```python
from build123d import *

# Parameters (mm, degrees)
PAD_DEPTH       = 22
BOX_W           = 28
BOX_H           = 44
BOX_DEPTH       = 11
SKETCH001_R     = 8.75
POCKET_DEPTH    = 33
FILLET_R        = 2
SKETCH003_R     = 3
POCKET002_DEPTH = 28.001


with BuildPart() as part:
    # Sketch → Pad (new body)
    with BuildSketch(Plane.XY):
        Polygon((0, 1), (17, 1), (17, 10), (17.5, 10), (17.5, 22), (15, 25), (2, 25), (-0.5, 22), (-0.5, 10), (0, 10), align=None)
    extrude(amount=PAD_DEPTH)

    # Box → Box (join)
    with BuildSketch(Plane(origin=(-5.5, -10, 22), x_dir=(1, 0, 0), z_dir=(0, 0, 1))):
        with Locations((14, 22)):
            Rectangle(BOX_W, BOX_H)
    extrude(amount=BOX_DEPTH)

    # Sketch001 (on Face4 of Box) → Pocket (cut)
    with BuildSketch(Plane(origin=(-5.5, -10, 0), x_dir=(1, 0, 0), z_dir=(0, 0, -1))):
        with Locations((14, -24.5)):
            Circle(SKETCH001_R)
    extrude(amount=-POCKET_DEPTH, mode=Mode.SUBTRACT)

    # Fillet
    fillet_edges = [part.edges().sort_by_distance(p)[0] for p in [
        (17.5, 22, 11),
        (15, 25, 11),
        (2, 25, 11),
        (17, 1, 11),
        (0, 1, 11),
        (-0.5, 22, 11),
    ]]
    fillet(fillet_edges, radius=FILLET_R)

    # Sketch003 (on Face23 of Fillet) → Pocket002 (cut, through all)
    with BuildSketch(Plane(origin=(22.5, -10, 22), x_dir=(0, 1, 0), z_dir=(1, 0, 0))):
        with Locations((7, 5.5)):
            Circle(SKETCH003_R)
        with Locations((37, 5.5)):
            Circle(SKETCH003_R)
    extrude(amount=-POCKET002_DEPTH, mode=Mode.SUBTRACT)


solid = part.part
```
Input: part model. Units: mm. Frame: model coordinates. A direction names the side the tool comes from. Give positions to 0.01 mm unless a question says otherwise; leave off trailing zeros. Write each loop counter-clockwise with the first axis right and the second up, starting at its lowest first coordinate (ties: lowest second). Pieces come first, ordered by that corner, then holes. Notation, with made-up numbers: (28, -37) - (69, -37) arc R19 cw to (69, -32) - close; hole circle Ø7 at (11, 21.25). An arc over 180 degrees is marked (long way). Write item = value, one per line. Start each with the question number.
1) Cut plane C-C (x = 8.5). Return loops of the section in (y, z), and give its area (3 significant figures).
2) Draft query along Z for faces 6 (the face through (8, 1, 11)), 7 (the face through (15, 7, 33)), 8 (the face through (8.7, -5.4, 25.7)). Return one class per face: pulls with the +Z half, pulls with the -Z half, needs draft (parallel to the pull), parting line crosses it, or undercut.
3) Material intervals for L1, parallel to Y at x = 8.5, z = 28; L2, parallel to Y at x = 8.5, z = 7; L3, parallel to Y at x = 21, z = 25.5, sorted ascending. Write a range as [from, to].
4) Reachability of faces 1 (the face through (16.328, 23.406, 10.846)), 2 (the face through (9, 25, 11)), 3 (the face through (-0.377, 21.966, 11.154)), 4 (the face through (-0.5, 16, 11)), 5 (the face through (17, 6, 11)) from +Z, -Z, +X, -X, +Y, -Y: full face, straight path, thin tool, end or side. Return the list, or none.
5) Cut plane D-D (x = 20). Return loops of the section in (y, z).
6) Pin query (flat end, axial travel): pin 1 (3.5 mm diameter, centred on x = 6.5, z = 11.5, fed in from +Y); pin 2 (0.6 mm diameter, centred on x = 0, z = 10.5, fed in from -Y); pin 3 (1.5 mm diameter, centred on x = 6, z = 21, fed in from -Y); pin 4 (5 mm diameter, centred on y = -3, z = 27.5, fed in from +X). Return the tip coordinate at first contact, or that it passes through.
7) Cut plane B-B (z = 27.5). Return loops of the section in (x, y), and give its area (3 significant figures).
8) Cut plane A-A (y = 27). Return loops of the section in (x, z), and give its area (3 significant figures).
Answers follow:
q1.outline = (-10, 22) - (1, 22) - (1, 0) - (5.75, 0) - (5.75, 33) - (-10, 33) - close; (23.25, 0) - (25, 0) - (25, 22) - (34, 22) - (34, 33) - (23.25, 33) - close; hole circle Ø6 at (-3, 27.5); hole circle Ø6 at (27, 27.5)
q1.area = 378 mm^2
q2.face_6 = needs draft
q2.face_7 = pulls with the +Z half
q2.face_8 = undercut
q3.L1 = [-10, -5.96], [-0.04, 5.75], [23.25, 24.04], [29.96, 34]
q3.L2 = [1, 5.75], [23.25, 25]
q3.L3 = [-10, -5.24], [-0.76, 24.76], [29.24, 34]
q4.face_1 = -Z, +X, +Y
q4.face_2 = -Z, +X, -X, +Y
q4.face_3 = -Z, -X, +Y
q4.face_4 = -Z, -X, +Y, -Y
q4.face_5 = -Z, +X, -Y
q5.outline = (-10, 22) - (34, 22) - (34, 33) - (-10, 33) - close; hole circle Ø6 at (-3, 27.5); hole circle Ø6 at (27, 27.5)
q6.pin_1 = 25
q6.pin_2 = 1.95
q6.pin_3 = 1
q6.pin_4 = through
q7.outline = (-5.5, -10) - (22.5, -10) - (22.5, -6) - (-5.5, -6) - close; (-5.5, 0) - (22.5, 0) - (22.5, 24) - (-5.5, 24) - close; (-5.5, 30) - (22.5, 30) - (22.5, 34) - (-5.5, 34) - close; hole circle Ø17.5 at (8.5, 14.5)
q7.area = 655 mm^2
q8.outline = (-5.5, 22) - (22.5, 22) - (22.5, 24.5) - (-5.5, 24.5) - close; (-5.5, 30.5) - (22.5, 30.5) - (22.5, 33) - (-5.5, 33) - close
q8.area = 140 mm^2
